from build123d import *

# Parameters (mm, degrees)
SKETCH1_W           = 18
SKETCH1_H           = 18
SKETCH1_R           = 1.5
SKETCH1_H_2         = 3
BOSS_EXTRUDE1_DEPTH = 2.5
SKETCH1_3_W         = 18
SKETCH1_3_H         = 3
BOSS_EXTRUDE2_DEPTH = 6
FILLET1_R           = 1.5


with BuildPart() as part:
    # Sketch1 → Boss-Extrude1 (new body)
    # profile 1 of 2: a face of its own
    with BuildSketch(Plane.XY):
        with Locations((0, 1.5)):
            Rectangle(SKETCH1_W, SKETCH1_H)
        with Locations((-5, 8)):
            Circle(SKETCH1_R, mode=Mode.SUBTRACT)
        with Locations((-0.5, 7)):
            Circle(SKETCH1_R, mode=Mode.SUBTRACT)
        with BuildLine():
            ThreePointArc((3.329179607, 6.658359214), (2.658359214, 8.670820393), (4.670820393, 9.341640786))
            Line((4.670820393, 9.341640786), (6.670820393, 8.341640786))
            ThreePointArc((6.670820393, 8.341640786), (7.275976213, 7.788596668), (7.5, 7))
            ThreePointArc((7.5, 7), (6.788596668, 5.724023787), (5.329179607, 5.658359214))
            Line((5.329179607, 5.658359214), (3.329179607, 6.658359214))
        make_face(mode=Mode.SUBTRACT)
    # profile 2 of 2: a face of its own
    with BuildSketch(Plane.XY):
        with Locations((0, -9)):
            Rectangle(SKETCH1_W, SKETCH1_H_2)
    extrude(amount=BOSS_EXTRUDE1_DEPTH)

    # Sketch1_3 → Boss-Extrude2 (add)
    with BuildSketch(Plane.XY):
        with Locations((0, -9)):
            Rectangle(SKETCH1_3_W, SKETCH1_3_H)
    extrude(amount=-BOSS_EXTRUDE2_DEPTH)

    # Fillet1
    fillet1_edges = [part.edges().sort_by_distance(p)[0] for p in [
        (0, -7.5, 0),
        (0, -10.5, 2.5),
    ]]
    fillet(fillet1_edges, radius=FILLET1_R)


solid = part.part
Read the model definition and answer for the solid it produces. Units are mm, in the model's axes. A direction names the side the tool comes from. Give positions to 0.01 mm unless a question says otherwise; leave off trailing zeros. Loops run counter-clockwise (first coordinate to the right, second up) from the corner with the lowest first, then second, coordinate; pieces in that order, holes last. Notation, with made-up numbers: (-3, -30.5) - (38, -30.5) arc R19 ccw to (38, -7.5) - close; hole circle Ø8 at (4.25, -31.75). An arc over 180 degrees is marked (long way). Answer as CSV lines item,"result". Start each with the question number.
1) Each of these flat-tipped pins is pushed along its axis until it touches: pin 1 Ø1 at (x, y) = (2.5, 5.5) entering from -Z; pin 2 Ø2 at (x, z) = (-2.5, -4) entering from +Y; pin 3 Ø2.5 at (x, y) = (-0.5, 7) entering from +Z. Where does it stop, or does it pass through?
2) Determine the mould class of faces 1 (the face through (0, 2, 0)), 2 (the face through (-0.825, 5.536, 1.232)), 3 (the face through (0.13, -10.05, 2.07)), 4 (the face through (0, -7.5, -4)) for opening direction Y: released by +Y, released by -Y, zero draft, split by the parting line, or undercut.
3) Find section B-B (y = 9). Write down the section's boundary in (x, z), then the cut area to 3 significant figures.
4) Find section C-C (x = -4.5). Write down the section's boundary in (y, z).
5) Straight lines are drawn through the part: L1, parallel to Z at x = 7.75, y = 4.25; L2, parallel to Y at x = -3.5, z = -4; L3, parallel to X at y = 6, z = 1. For each, find the intervals that lie inside material, in ascending order. Write a range as from..to.
6) Which of the six approach directions +Z, -Z, +X, -X, +Y, -Y give full straight-line access (tool end or side, diameter ignored) to faces 5 (the face through (4.343, 6.151, 1.232)), 6 (the face through (0.13, -7.05, -0.43))?
7) Find section A-A (x = -0.5). Write down the section's boundary in (y, z), then the cut area to 3 significant figures.
8) Find section D-D (z = -4). Write down the section's boundary in (x, y).
Findings below:
1,pin 1,"z = 0"
1,pin 2,"y = -7.5"
1,pin 3,"through"
2,face 1,"zero draft"
2,face 2,"undercut"
2,face 3,"released by -Y"
2,face 4,"released by +Y"
3,outline,"(-9, 0) - (-6.12, 0) - (-6.12, 2.5) - (-9, 2.5) - close; (-3.88, 0) - (2.88, 0) - (2.88, 2.5) - (-3.88, 2.5) - close; (5.35, 0) - (9, 0) - (9, 2.5) - (5.35, 2.5) - close"
3,area,"33.2 mm^2"
4,outline,"(-10.5, -6) - (-7.5, -6) - (-7.5, -1.5) arc R1.5 cw to (-6, 0) - (6.59, 0) - (6.59, 2.5) - (-9, 2.5) arc R1.5 ccw to (-10.5, 1) - close; (9.41, 0) - (10.5, 0) - (10.5, 2.5) - (9.41, 2.5) - close"
5,L1,"0..2.5"
5,L2,"-10.5..-7.5"
5,L3,"-9..-1.62, 0.62..4.65, 7.12..9"
6,face 5,"+Z, -Z"
6,face 6,"-Z, +X, -X, +Y"
7,outline,"(-10.5, -6) - (-7.5, -6) - (-7.5, -1.5) arc R1.5 cw to (-6, 0) - (5.5, 0) - (5.5, 2.5) - (-9, 2.5) arc R1.5 ccw to (-10.5, 1) - close; (8.5, 0) - (10.5, 0) - (10.5, 2.5) - (8.5, 2.5) - close"
7,area,"63.0 mm^2"
8,outline,"(-9, -10.5) - (9, -10.5) - (9, -7.5) - (-9, -7.5) - close"
